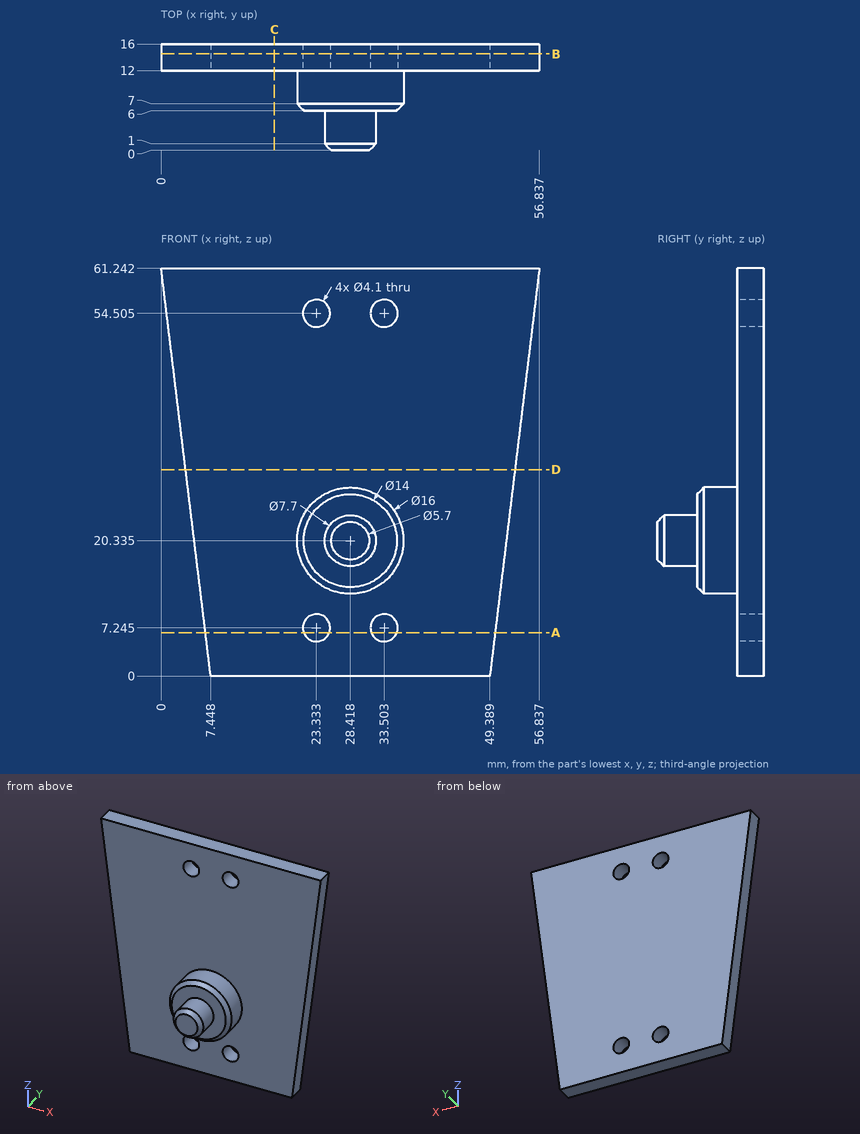
Geometry: see drawing. Coordinates: mm, zero at the bounding-box minimum. Round coordinates to 2 decimals unless told otherwise and drop trailing zeros. Write each loop counter-clockwise with the first axis right and the second up, starting at its lowest first coordinate (ties: lowest second). Pieces come first, ordered by that corner, then holes. Notation, with made-up numbers: (51.5, 20.25) - (67.5, 20.25) arc R30 ccw to (67.5, 51.25) - close; hole circle Ø6 at (38, 88). An arc over 180 degrees is marked (long way). Use CSV: the item, a comma, the result in double quotes. Start each with the question number.
(1) Cut plane B-B, the plane y = 14.5. Give the number of separate pieces and of enclosed holes in the cut face, and give its area (3 significant figures).
(2) Material intervals for probe 1 along Z at (x, y) = (35, 12.75) (1 decimal); probe 2 along Y at (x, z) = (19, 48.5); probe 3 along X at (y, z) = (11.5, 24.5), sorted ascending. Write a range as [from, to].
(3) Cut plane A-A, the plane z = 6.5. Return loops of the section in (x, y).
(4) Cut plane D-D, the plane z = 31. Return loops of the section in (x, y).
(5) First-contact query: pin 1 Ø3 at (x, y) = (28.5, 2.5) entering from -Z (1 decimal); pin 2 Ø6 at (y, z) = (11.5, 45) entering from +X; pin 3 Ø3 at (x, z) = (13, 18.5) entering from -Y; pin 4 Ø2.5 at (x, z) = (23.33, 7.25) entering from -Y. Flat tips, straight axial feed; report the tip coordinate or a pass-through.
(6) Cut plane C-C, the plane x = 17. Return loops of the section in (y, z).
Geometry says:
1,separate pieces,"1"
1,enclosed holes,"4"
1,area,"2,970 mm²"
2,probe 1,"[0, 5.8], [8.6, 53.1], [55.9, 61.2]"
2,probe 2,"[12, 16]"
2,probe 3,"[21.59, 35.25]"
3,outline,"(6.66, 12) - (21.42, 12) - (21.42, 16) - (6.66, 16) - close; (25.24, 12) - (31.59, 12) - (31.59, 16) - (25.24, 16) - close; (35.41, 12) - (50.18, 12) - (50.18, 16) - (35.41, 16) - close"
4,outline,"(3.68, 12) - (53.16, 12) - (53.16, 16) - (3.68, 16) - close"
5,pin 1,"z = 16.5"
5,pin 2,"x = 55.22"
5,pin 3,"y = 12"
5,pin 4,"through"
6,outline,"(12, 0) - (16, 0) - (16, 61.24) - (12, 61.24) - close"
